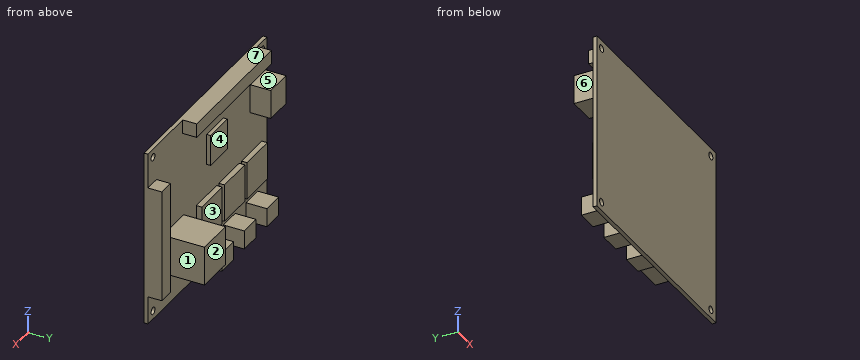
```python
from build123d import *

# Parameters (mm, degrees)
SKETCH1_W                 = 100.33
SKETCH1_H                 = 80.01
BOSS_EXTRUDE1_DEPTH       = 1.778
F_4_CLEARANCE_HOLE1_D     = 3.2639
F_4_CLEARANCE_HOLE1_DEPTH = 12.7
F_4_CLEARANCE_HOLE1_TIP   = 0.980574487
SKETCH4_W                 = 17.145
SKETCH4_H                 = 17.145
BOSS_EXTRUDE2_DEPTH       = 2.54
SKETCH6_W                 = 9.906
SKETCH6_H                 = 8.509
BOSS_EXTRUDE3_DEPTH       = 9.525
LPATTERN1_COUNT           = 3
LPATTERN1_PITCH           = 19.05
SKETCH7_W                 = 14.097
SKETCH7_H                 = 14.097
BOSS_EXTRUDE4_DEPTH       = 1.778
SKETCH8_W                 = 62.992
SKETCH8_H                 = 6.35
BOSS_EXTRUDE5_DEPTH       = 6.35
SKETCH9_W                 = 7.270390316
SKETCH9_H                 = 51.271334807
BOSS_EXTRUDE6_DEPTH       = 6.35
SKETCH10_W                = 17.620008018
SKETCH10_H                = 17.836647461
BOSS_EXTRUDE7_DEPTH       = 19.05
SKETCH11_W                = 12.792637694
SKETCH11_H                = 13.15401164
BOSS_EXTRUDE8_DEPTH       = 9.525


with BuildPart() as part:
    # Sketch1 → Boss-Extrude1 (new body)
    with BuildSketch(Plane(origin=(0, 0, 0), x_dir=(1, 0, 0), z_dir=(0, 1, 0))):
        Rectangle(SKETCH1_W, SKETCH1_H)
    extrude(amount=BOSS_EXTRUDE1_DEPTH)

    # #4 Clearance Hole1
    with Locations(Plane(origin=(0, 1.778, 0), x_dir=(1, 0, 0), z_dir=(0, 1, 0))):
        with Locations((-46.355, 36.195), (45.847, -36.195), (-46.355, -36.195), (45.847, 36.195)):
            Hole(F_4_CLEARANCE_HOLE1_D / 2, depth=F_4_CLEARANCE_HOLE1_DEPTH)
            with Locations((0, 0, -(F_4_CLEARANCE_HOLE1_DEPTH + F_4_CLEARANCE_HOLE1_TIP / 2))):  # 118° drill point
                Cone(0, F_4_CLEARANCE_HOLE1_D / 2, F_4_CLEARANCE_HOLE1_TIP, mode=Mode.SUBTRACT)

    # Sketch4 → Boss-Extrude2 (add)
    with BuildSketch(Plane(origin=(0, 1.778, 0), x_dir=(1, 0, 0), z_dir=(0, 1, 0))):
        with Locations((-37.2745, 15.1765)):
            Rectangle(SKETCH4_W, SKETCH4_H)
    boss_extrude2 = extrude(amount=BOSS_EXTRUDE2_DEPTH)

    # Sketch6 → Boss-Extrude3 (add)
    with BuildSketch(Plane(origin=(0, 1.778, 0), x_dir=(1, 0, 0), z_dir=(0, 1, 0))):
        with Locations((-37.465, 32.5755)):
            Rectangle(SKETCH6_W, SKETCH6_H)
    boss_extrude3 = extrude(amount=BOSS_EXTRUDE3_DEPTH)

    # LPattern1: Boss-Extrude2, Boss-Extrude3 ×3
    with Locations(*[(i * LPATTERN1_PITCH, 0, 0) for i in range(1, LPATTERN1_COUNT)]):
        add(boss_extrude2)
        add(boss_extrude3)

    # Sketch7 → Boss-Extrude4 (add)
    with BuildSketch(Plane(origin=(0, 1.778, 0), x_dir=(1, 0, 0), z_dir=(0, 1, 0))):
        with Locations((-6.4135, -15.0495)):
            Rectangle(SKETCH7_W, SKETCH7_H)
    extrude(amount=BOSS_EXTRUDE4_DEPTH)

    # Sketch8 → Boss-Extrude5 (add)
    with BuildSketch(Plane(origin=(0, 1.778, 0), x_dir=(1, 0, 0), z_dir=(0, 1, 0))):
        with Locations((-10.668, -36.83)):
            Rectangle(SKETCH8_W, SKETCH8_H)
    extrude(amount=BOSS_EXTRUDE5_DEPTH)

    # Sketch9 → Boss-Extrude6 (add)
    with BuildSketch(Plane(origin=(0, 1.778, 0), x_dir=(1, 0, 0), z_dir=(0, 1, 0))):
        with Locations((46.529804842, 1.552582673)):
            Rectangle(SKETCH9_W, SKETCH9_H)
    extrude(amount=BOSS_EXTRUDE6_DEPTH)

    # Sketch10 → Boss-Extrude7 (add)
    with BuildSketch(Plane(origin=(0, 1.778, 0), x_dir=(1, 0, 0), z_dir=(0, 1, 0))):
        with Locations((28.957472194, 13.93713749)):
            Rectangle(SKETCH10_W, SKETCH10_H)
    extrude(amount=BOSS_EXTRUDE7_DEPTH)

    # Sketch11 → Boss-Extrude8 (add)
    with BuildSketch(Plane(origin=(0, 1.778, 0), x_dir=(1, 0, 0), z_dir=(0, 1, 0))):
        with Locations((-42.172339514, -18.972132172)):
            Rectangle(SKETCH11_W, SKETCH11_H)
    extrude(amount=BOSS_EXTRUDE8_DEPTH)


solid = part.part
```
Input: part model. Units: mm. Frame: model coordinates. Face numbers are marked on the shaded views. A direction names the side the tool comes from. Round coordinates to 2 decimals unless told otherwise and drop trailing zeros. Loops run counter-clockwise (first coordinate to the right, second up) from the corner with the lowest first, then second, coordinate; pieces in that order, holes last. Notation, with made-up numbers: (54, -10) -> (112, -10) arc R23 ccw to (112, 22) -> close; hole circle Ø6 at (-29, 45). An arc over 180 degrees is marked (long way). Use one line per item in the form item = value. Start each with the question number.
Item 1: Section query A-A on x = 30.5. Return the cut outline in (y, z) (3 decimals), then the cut area to 3 significant figures.
Item 2: Mould query, pull axis Z, two halves, no side actions, for the marked faces 5, 6 and 7. Classes: pulls with the +Z half, pulls with the -Z half, needs draft (parallel to the pull), parting line crosses it, or undercut.
Item 3: Section query D-D on y = 18.25. Return the cut outline in (x, z).
Item 4: Set-up query: the marked faces 1, 2, 3 and 4. Return all of +Z, -Z, +X, -X, +Y, -Y with unobstructed straight access to the full face (end or side cutting, diameter ignored); none if empty.
Item 5: Section query B-B on z = -19. Return the cut outline in (x, y) (3 decimals).
Item 6: Contact query for flat-ended pins moving along their axis: pin 1 Ø2 at (y, z) = (3, 18) entering from -X; pin 2 Ø2.5 at (x, z) = (-1.5, -33) entering from +Y; pin 3 Ø4 at (x, z) = (45.847, -36.195) entering from +Y; pin 4 Ø7 at (y, z) = (5, -32.5) entering from +X (3 decimals). Output: stop coordinate, or through.
Item 7: Section query C-C on x = -2. Return the cut outline in (y, z) (3 decimals).
Item 8: Material intervals for L1, parallel to Z at x = -18, y = 4.75 (3 decimals); L2, parallel to X at y = 12.25, z = -11.5; L3, parallel to Y at x = -16, z = 17.5, sorted ascending. Write a range as from..to.
Ans:
q1.outline = (0, -40.005) -> (1.778, -40.005) -> (1.778, -22.855) -> (20.828, -22.855) -> (20.828, -5.019) -> (1.778, -5.019) -> (1.778, 40.005) -> (0, 40.005) -> close
q1.area = 482 mm^2
q2.face_5 = undercut
q2.face_6 = needs draft
q2.face_7 = pulls with the +Z half
q3.outline = (20.15, -22.86) -> (37.77, -22.86) -> (37.77, -5.02) -> (20.15, -5.02) -> close
q4.face_1 = +Z, -Z, +Y
q4.face_2 = +Z, -Z, +X, -X, +Y
q4.face_3 = -X, +Y
q4.face_4 = +Y
q5.outline = (-50.165, 0) -> (50.165, 0) -> (50.165, 8.128) -> (42.895, 8.128) -> (42.895, 1.778) -> (37.767, 1.778) -> (37.767, 20.828) -> (20.147, 20.828) -> (20.147, 1.778) -> (9.398, 1.778) -> (9.398, 4.318) -> (-7.747, 4.318) -> (-7.747, 1.778) -> (-9.652, 1.778) -> (-9.652, 4.318) -> (-26.797, 4.318) -> (-26.797, 1.778) -> (-28.702, 1.778) -> (-28.702, 4.318) -> (-45.847, 4.318) -> (-45.847, 1.778) -> (-50.165, 1.778) -> close
q6.pin_1 = -48.57
q6.pin_2 = 11.3
q6.pin_3 = 1.78
q6.pin_4 = 50.165
q7.outline = (0, -40.005) -> (1.778, -40.005) -> (1.778, -36.83) -> (11.303, -36.83) -> (11.303, -28.321) -> (1.778, -28.321) -> (1.778, -23.749) -> (4.318, -23.749) -> (4.318, -6.604) -> (1.778, -6.604) -> (1.778, 8.001) -> (3.556, 8.001) -> (3.556, 22.098) -> (1.778, 22.098) -> (1.778, 33.655) -> (8.128, 33.655) -> (8.128, 40.005) -> (0, 40.005) -> close
q8.L1 = -36.83..-28.321, 33.655..40.005
q8.L2 = 20.15..37.77
q8.L3 = 0..1.78
